Work out the finished part from the listing and answer in its coordinate system (mm). Give positions to 0.01 mm unless a question says otherwise; leave off trailing zeros. Loops run counter-clockwise (first coordinate to the right, second up) from the corner with the lowest first, then second, coordinate; pieces in that order, holes last. Notation, with made-up numbers: (-21.75, 25) - (34.25, 25) arc R19 cw to (34.25, 38) - close; hole circle Ø8 at (15, -26). An arc over 180 degrees is marked (long way). One line per question, with ' | ' between items. Start each with the question number.
1. Section D-D (y = -18.5) is taken. Determine the outline of the cut face in (x, z), plus the area to 3 significant figures.
2. Section C-C (z = 5.35) is taken. Determine the outline of the cut face in (x, y).
3. For a pull along Y with two mould halves and no side action, classify faces 1 (the face through (10.2, 21, 5.5)), 2 (the face through (27.292, 20.086, 5.493)), 3 (the face through (-7.708, 20.086, 5.493)), 4 (the face through (-11.5, -0.3, 5.5)) as released by +Y, released by -Y, zero draft, split by the parting line, or undercut.
4. Find the intervals of material crossed by line 1 (Y direction, x = 27.5, z = 5.35); line 2 (X direction, y = 18.5, z = 5.35); line 3 (Y direction, x = 0, z = 5.6), in increasing order.
5. Section A-A (x = 0) is taken. Determine the outline of the cut face in (y, z).
6. This flat-tipped pin is pushed along its axis until it touches: pin 1 (2.5 mm diameter, centred on x = 27.5, y = -18.5, fed in from -Z). Where does it stop, or does it pass through?
7. Section B-B (y = 0) is taken. Determine the outline of the cut face in (x, z), plus the area to 3 significant figures.
from build123d import *

# Parameters (mm, degrees)
CYLINDER034_R     = 1.6
CYLINDER034_DEPTH = 10
CYLINDER035_R     = 1.6
CYLINDER035_DEPTH = 10
CYLINDER036_R     = 1.6
CYLINDER036_DEPTH = 10
CYLINDER037_R     = 1.6
CYLINDER037_DEPTH = 10
CYLINDER038_R     = 2
CYLINDER038_DEPTH = 10
BOX011_W          = 44
BOX011_H          = 42
BOX011_DEPTH      = 1


with BuildPart() as cylinder034:
    # Cylinder034 → Cylinder034 (new body)
    with BuildSketch(Plane(origin=(-7.5, -18.5, 0), x_dir=(1, 0, 0), z_dir=(0, 0, 1))):
        Circle(CYLINDER034_R)
    extrude(amount=CYLINDER034_DEPTH)


with BuildPart() as cylinder035:
    # Cylinder035 → Cylinder035 (new body)
    with BuildSketch(Plane(origin=(-7.5, 18.5, 0), x_dir=(1, 0, 0), z_dir=(0, 0, 1))):
        Circle(CYLINDER035_R)
    extrude(amount=CYLINDER035_DEPTH)


with BuildPart() as cylinder036:
    # Cylinder036 → Cylinder036 (new body)
    with BuildSketch(Plane(origin=(27.5, -18.5, 0), x_dir=(1, 0, 0), z_dir=(0, 0, 1))):
        Circle(CYLINDER036_R)
    extrude(amount=CYLINDER036_DEPTH)


with BuildPart() as cylinder037:
    # Cylinder037 → Cylinder037 (new body)
    with BuildSketch(Plane(origin=(27.5, 18.5, 0), x_dir=(1, 0, 0), z_dir=(0, 0, 1))):
        Circle(CYLINDER037_R)
    extrude(amount=CYLINDER037_DEPTH)


with BuildPart() as fusion021:
    # Cylinder038 → Cylinder038 (new body)
    with BuildSketch(Plane.XY):
        Circle(CYLINDER038_R)
    extrude(amount=CYLINDER038_DEPTH)

    # Fusion021: union Cylinder034, Cylinder035, Cylinder036, Cylinder037
    add(cylinder034.part)
    add(cylinder035.part)
    add(cylinder036.part)
    add(cylinder037.part)


with BuildPart() as copperplate:
    # Box011 → Box011 (new body)
    with BuildSketch(Plane(origin=(-11.5, -21, 1), x_dir=(1, 0, 0), z_dir=(0, 0, 1))):
        with Locations((22, 21)):
            Rectangle(BOX011_W, BOX011_H)
    extrude(amount=BOX011_DEPTH)

    # Cut010: cut Fusion021
    add(fusion021.part, mode=Mode.SUBTRACT)


with BuildPart() as copperplate_1:
    # Cut010 placement: moved
    add(copperplate.part.moved(Location((0, 0, 4))))


solid = copperplate_1.part
Conclusion:
1) outline: (-11.5, 5) - (-9.1, 5) - (-9.1, 6) - (-11.5, 6) - close; (-5.9, 5) - (25.9, 5) - (25.9, 6) - (-5.9, 6) - close; (29.1, 5) - (32.5, 5) - (32.5, 6) - (29.1, 6) - close | area: 37.6 mm²
2) outline: (-11.5, -21) - (32.5, -21) - (32.5, 21) - (-11.5, 21) - close; hole circle Ø3.2 at (-7.5, -18.5); hole circle Ø3.2 at (-7.5, 18.5); hole circle Ø4 at (0, 0); hole circle Ø3.2 at (27.5, -18.5); hole circle Ø3.2 at (27.5, 18.5)
3) face 1: released by +Y | face 2: undercut | face 3: undercut | face 4: zero draft
4) line 1: -21 to -20.1, -16.9 to 16.9, 20.1 to 21 | line 2: -11.5 to -9.1, -5.9 to 25.9, 29.1 to 32.5 | line 3: -21 to -2, 2 to 21
5) outline: (-21, 5) - (-2, 5) - (-2, 6) - (-21, 6) - close; (2, 5) - (21, 5) - (21, 6) - (2, 6) - close
6) pin 1: through
7) outline: (-11.5, 5) - (-2, 5) - (-2, 6) - (-11.5, 6) - close; (2, 5) - (32.5, 5) - (32.5, 6) - (2, 6) - close | area: 40.0 mm²
